```python
from build123d import *

# Parameters (mm, degrees)
SKETCH_1_W      = 81
SKETCH_1_H      = 90
EXTRUDE_1_DEPTH = 5.6
SKETCH_2_W      = 15.8
SKETCH_2_H      = 20
SKETCH_2_R      = 1.6
EXTRUDE_2_DEPTH = 5.6
FILLET_1_R      = 2


with BuildPart() as part:
    # ｽｹｯﾁ1 → ﾎﾞｽ - 押し出し1 (new body)
    with BuildSketch(Plane(origin=(0, 0, 0), x_dir=(1, 0, 0), z_dir=(0, 1, 0))):
        Rectangle(SKETCH_1_W, SKETCH_1_H)
    extrude(amount=EXTRUDE_1_DEPTH)

    # ｽｹｯﾁ2 → ﾎﾞｽ - 押し出し2 (add)
    # profile 1 of 4: a face of its own
    with BuildSketch(Plane(origin=(0, 5.6, 0), x_dir=(1, 0, 0), z_dir=(0, 1, 0))):
        with Locations((-48.4, 17.5)):
            Rectangle(SKETCH_2_W, SKETCH_2_H)
        with Locations(Location((-51.3, 17.5, 0), (0, 0, 270))):
            Circle(SKETCH_2_R, mode=Mode.SUBTRACT)
    # profile 2 of 4: a face of its own
    with BuildSketch(Plane(origin=(0, 5.6, 0), x_dir=(1, 0, 0), z_dir=(0, 1, 0))):
        with Locations((48.4, 17.5)):
            Rectangle(SKETCH_2_W, SKETCH_2_H)
        with Locations(Location((51.3, 17.5, 0), (0, 0, 90))):
            Circle(SKETCH_2_R, mode=Mode.SUBTRACT)
    # profile 3 of 4: a face of its own
    with BuildSketch(Plane(origin=(0, 5.6, 0), x_dir=(1, 0, 0), z_dir=(0, 1, 0))):
        with Locations((-48.4, -17.5)):
            Rectangle(SKETCH_2_W, SKETCH_2_H)
        with Locations(Location((-51.3, -17.5, 0), (0, 0, 90))):
            Circle(SKETCH_2_R, mode=Mode.SUBTRACT)
    # profile 4 of 4: a face of its own
    with BuildSketch(Plane(origin=(0, 5.6, 0), x_dir=(1, 0, 0), z_dir=(0, 1, 0))):
        with Locations((48.4, -17.5)):
            Rectangle(SKETCH_2_W, SKETCH_2_H)
        with Locations(Location((51.3, -17.5, 0), (0, 0, 270))):
            Circle(SKETCH_2_R, mode=Mode.SUBTRACT)
    extrude(amount=-EXTRUDE_2_DEPTH)

    # ﾌｨﾚｯﾄ1
    fillet_1_edges = [part.edges().sort_by_distance(p)[0] for p in [
        (56.3, 2.8, -27.5),
        (56.3, 2.8, -7.5),
        (-56.3, 2.8, -27.5),
        (-56.3, 2.8, -7.5),
        (-56.3, 2.8, 27.5),
        (-56.3, 2.8, 7.5),
        (56.3, 2.8, 27.5),
        (56.3, 2.8, 7.5),
        (40.5, 2.8, 45),
        (-40.5, 2.8, 45),
        (-40.5, 2.8, -45),
        (40.5, 2.8, -45),
    ]]
    fillet(fillet_1_edges, radius=FILLET_1_R)


solid = part.part
```
Part model, mm, in its own coordinate system. A direction names the side the tool comes from. Give positions to 0.01 mm unless a question says otherwise; leave off trailing zeros. Write each loop counter-clockwise with the first axis right and the second up, starting at its lowest first coordinate (ties: lowest second). Pieces come first, ordered by that corner, then holes. Notation, with made-up numbers: (-20, -26.75) -> (34, -26.75) arc R25 cw to (34, 10.25) -> close; hole circle Ø8 at (42.25, 59). An arc over 180 degrees is marked (long way). Put each result on its own line as item: value. Start each with the question number.
Item 1: Cut at B-B (x = -51.3). List the corners of the cut face in (y, z), then the cut area to 3 significant figures.
Item 2: Pull direction X, two halves, no side cores. Call faces 1 (the face through (-56.3, 3, 18)), 2 (the face through (-47, 3, -27.5)), 3 (the face through (50.33, 2.84, 16.23)): pulls with the +X half, pulls with the -X half, needs draft (parallel to the pull), parting line crosses it, or undercut.
Item 3: Cut at D-D (y = 3.4). State how many separate pieces and enclosed holes the cut face has, then the cut area to 3 significant figures.
Item 4: Which spindle directions (+Z, -Z, +X, -X, +Y, -Y) get a long thin tool onto all of the face, cutting with end or side? Do faces 4 (the face through (-40.5, 3, 35)), 5 (the face through (-47, 3, -7.5)), 6 (the face through (47, 3, -7.5)), 7 (the face through (47, 3, -27.5)). Say none if no direction does.
Item 5: Pin check, flat tips, straight feed: pin 1 Ø1.7 at (x, y) = (49, 4) entering from +Z; pin 2 Ø3 at (y, z) = (3.5, 2) entering from +X; pin 3 Ø1.7 at (y, z) = (4, 35.5) entering from -X. Stop position of each tip, or through.
Item 6: Wall check: L1, parallel to X at y = 3.15, z = 17.5; L2, parallel to Z at x = 49.5, y = 2.1; L3, parallel to X at y = 3.4, z = 18.5. Give the ranges that are in metal, low to high. Write a range as [from, to].
Item 7: Cut at C-C (z = -17.5). List the corners of the cut face in (x, y), then the cut area to 3 significant figures.
Item 8: Cut at A-A (x = 42.5). List the corners of the cut face in (y, z).
Answer list:
1. outline: (0, -27.5) -> (5.6, -27.5) -> (5.6, -19.1) -> (0, -19.1) -> close; (0, -15.9) -> (5.6, -15.9) -> (5.6, -7.5) -> (0, -7.5) -> close; (0, 7.5) -> (5.6, 7.5) -> (5.6, 15.9) -> (0, 15.9) -> close; (0, 19.1) -> (5.6, 19.1) -> (5.6, 27.5) -> (0, 27.5) -> close
1. area: 188 mm2
2. face 1: pulls with the -X half
2. face 2: needs draft
2. face 3: undercut
3. separate pieces: 1
3. enclosed holes: 4
3. area: 8,510 mm2
4. face 4: +Z, -X, +Y, -Y
4. face 5: -X, +Y, -Y
4. face 6: +X, +Y, -Y
4. face 7: -Z, +X, +Y, -Y
5. pin 1: stops at z = 27.5
5. pin 2: stops at x = 40.5
5. pin 3: stops at x = -40.5
6. L1: x = [-56.3, -52.9], [-49.7, 49.7], [52.9, 56.3]
6. L2: z = [-27.5, -7.5], [7.5, 27.5]
6. L3: x = [-56.3, -52.55], [-50.05, 50.05], [52.55, 56.3]
7. outline: (-56.3, 0) -> (-52.9, 0) -> (-52.9, 5.6) -> (-56.3, 5.6) -> close; (-49.7, 0) -> (49.7, 0) -> (49.7, 5.6) -> (-49.7, 5.6) -> close; (52.9, 0) -> (56.3, 0) -> (56.3, 5.6) -> (52.9, 5.6) -> close
7. area: 595 mm2
8. outline: (0, -27.5) -> (5.6, -27.5) -> (5.6, -7.5) -> (0, -7.5) -> close; (0, 7.5) -> (5.6, 7.5) -> (5.6, 27.5) -> (0, 27.5) -> close
